from build123d import *

# Parameters (mm, degrees)
ESQUISSE1_R        = 1.75
BOSS_EXTRU_1_DEPTH = 4
ESQUISSE3_R        = 3.1
BOSS_EXTRU_2_DEPTH = 0.75
ESQUISSE4_R        = 1.75
BOSS_EXTRU_3_DEPTH = 2.6
ESQUISSE5_R        = 3.1
BOSS_EXTRU_4_DEPTH = 0.75
ESQUISSE6_R        = 1.75
BOSS_EXTRU_5_DEPTH = 3.3
CHANFREIN1_SIZE    = 1.5
CONG_1_R           = 1.75


with BuildPart() as part:
    # Esquisse1 → Boss.-Extru.1 (new body)
    with BuildSketch(Plane.XY):
        Circle(ESQUISSE1_R)
    extrude(amount=BOSS_EXTRU_1_DEPTH)

    # Esquisse3 → Boss.-Extru.2 (add)
    with BuildSketch(Plane(origin=(0, 0, 0), x_dir=(-1, 0, 0), z_dir=(0, 0, -1))):
        Circle(ESQUISSE3_R)
    extrude(amount=BOSS_EXTRU_2_DEPTH)

    # Esquisse4 → Boss.-Extru.3 (add)
    with BuildSketch(Plane(origin=(0, 0, -0.75), x_dir=(-1, 0, 0), z_dir=(0, 0, -1))):
        Circle(ESQUISSE4_R)
    extrude(amount=BOSS_EXTRU_3_DEPTH)

    # Esquisse5 → Boss.-Extru.4 (add)
    with BuildSketch(Plane(origin=(0, 0, -3.35), x_dir=(-1, 0, 0), z_dir=(0, 0, -1))):
        Circle(ESQUISSE5_R)
    extrude(amount=BOSS_EXTRU_4_DEPTH)

    # Esquisse6 → Boss.-Extru.5 (add)
    with BuildSketch(Plane(origin=(0, 0, -4.1), x_dir=(-1, 0, 0), z_dir=(0, 0, -1))):
        Circle(ESQUISSE6_R)
    extrude(amount=BOSS_EXTRU_5_DEPTH)

    # Chanfrein1
    chanfrein1_edges = [part.edges().sort_by_distance(p)[0] for p in [
        (-1.75, 0, 4),
    ]]
    chamfer(chanfrein1_edges, length=CHANFREIN1_SIZE)

    # Congé1
    cong_1_edges = [part.edges().sort_by_distance(p)[0] for p in [
        (1.75, 0, -7.4),
    ]]
    fillet(cong_1_edges, radius=CONG_1_R)


solid = part.part
Geometry: final body of the model. Coordinates: model frame, mm. A direction names the side the tool comes from. Give positions to 0.01 mm unless a question says otherwise; leave off trailing zeros. Write each loop counter-clockwise with the first axis right and the second up, starting at its lowest first coordinate (ties: lowest second). Pieces come first, ordered by that corner, then holes. Notation, with made-up numbers: (22.5, 46.5) - (62.5, 46.5) arc R32 ccw to (62.5, 75.5) - close; hole circle Ø9 at (-10, 40). An arc over 180 degrees is marked (long way). Return JSON: item names as keys, results as strings. Group by question number.
1) First-contact query: P1, Ø2, axis at y = 2.5, z = -1.5, coming from the +X side; P2, Ø2, axis at x = -2.5, y = -2, coming from the -Z side; P3, Ø3, axis at y = 2.5, z = -6, coming from the -X side; P4, Ø1.9, axis at x = 0, y = 1, coming from the -Z side. Flat tips, straight axial feed; report the tip coordinate or a pass-through.
2) Mould query, pull axis Z, two halves, no side actions, for faces 4 (the conical face through (-0.11, -0.48, 3.76)), 5 (the flat face through (-2, 0, -3.35)), 6 (the cylindrical face through (-1.617, -0.67, -4.864)). Classes: released by +Z, released by -Z, zero draft, split by the parting line, or undercut.
3) Line query: line 1 (Z direction, x = -2.5, y = -0.75); line 2 (Z direction, x = -0.75, y = -0.25); line 3 (X direction, y = 0.75, z = -2.5). Output: solid intervals per line, ascending.
4) Section A-A on x = 0. Return the cut outline in (y, z).
5) Section B-B on y = -2. Return the cut outline in (x, z), plus the area to 3 significant figures.
6) Section D-D on x = 2.25. Return the cut outline in (y, z).
7) Set-up query: faces 1 (the flat face through (-2, 0, 0)), 2 (the flat face through (-2, 0, -4.1)), 3 (the cylindrical face through (-1.617, -0.67, -2.032)). Return all of +Z, -Z, +X, -X, +Y, -Y with unobstructed straight access to the full face (end or side cutting, diameter ignored); none if empty.
Filled in:
{
 "1": {"P1": "stops at x = 2.5", "P2": "stops at z = -4.1", "P3": "stops at x = -1.42", "P4": "stops at z = -7.4"},
 "2": {"face 4": "released by +Z", "face 5": "undercut", "face 6": "zero draft"},
 "3": {"line 1": "z = -4.1 to -3.35, -0.75 to 0", "line 2": "z = -7.21 to 3.46", "line 3": "x = -1.58 to 1.58"},
 "4": {"outline": "(-3.1, -4.1) - (-1.75, -4.1) - (-1.75, -5.65) arc R1.75 ccw to (1.75, -5.65) - (1.75, -4.1) - (3.1, -4.1) - (3.1, -3.35) - (1.75, -3.35) - (1.75, -0.75) - (3.1, -0.75) - (3.1, 0) - (1.75, 0) - (1.75, 2.5) - (0.25, 4) - (-0.25, 4) - (-1.75, 2.5) - (-1.75, 0) - (-3.1, 0) - (-3.1, -0.75) - (-1.75, -0.75) - (-1.75, -3.35) - (-3.1, -3.35) - close"},
 "5": {"outline": "(-2.37, -4.1) - (2.37, -4.1) - (2.37, -3.35) - (-2.37, -3.35) - close; (-2.37, -0.75) - (2.37, -0.75) - (2.37, 0) - (-2.37, 0) - close", "area": "7.11 mm^2"},
 "6": {"outline": "(-2.13, -4.1) - (2.13, -4.1) - (2.13, -3.35) - (-2.13, -3.35) - close; (-2.13, -0.75) - (2.13, -0.75) - (2.13, 0) - (-2.13, 0) - close"},
 "7": {"face 1": "+Z", "face 2": "-Z", "face 3": "none"}
}
